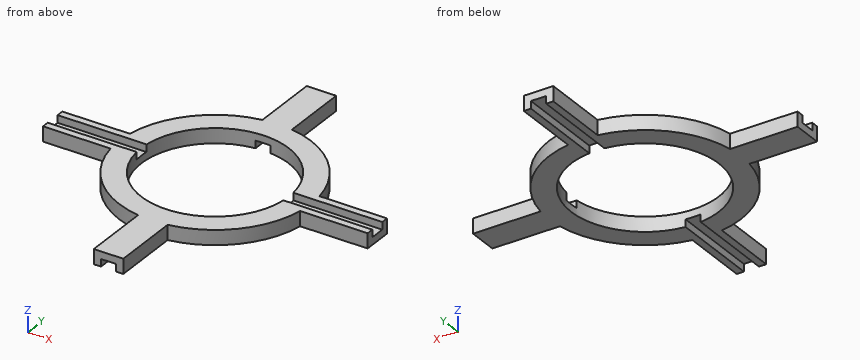
```python
from build123d import *

# Parameters (mm, degrees)
SKETCH1_R                    = 26
SKETCH1_R_2                  = 20
RELIEVED_FLOATING_RING_DEPTH = 4
SKETCH2_W                    = 20
SKETCH2_H                    = 8
X_SLIDE_PAD_1_DEPTH          = 4
SKETCH3_W                    = 8
SKETCH3_H                    = 20
Y_SLIDE_PAD_1_DEPTH          = 4
SKETCH4_W                    = 20
SKETCH4_H                    = 8
X_SLIDE_PAD_1_2_DEPTH        = 4
SKETCH5_W                    = 8
SKETCH5_H                    = 20
Y_SLIDE_PAD_1_2_DEPTH        = 4
SKETCH6_W                    = 4.1
SKETCH6_H                    = 90
LOWER_Y_SLOTS_W4P1_H2_DEPTH  = 2
SKETCH7_W                    = 90
SKETCH7_H                    = 4.1
UPPER_X_SLOTS_W4P1_H2_DEPTH  = 2


with BuildPart() as part:
    # Sketch1 → Relieved_Floating_Ring (new body)
    with BuildSketch(Plane.XY):
        Circle(SKETCH1_R)
        Circle(SKETCH1_R_2, mode=Mode.SUBTRACT)
    extrude(amount=RELIEVED_FLOATING_RING_DEPTH)

    # Sketch2 → X_Slide_Pad_-1 (add)
    with BuildSketch(Plane.XY):
        with Locations((-34, 0)):
            Rectangle(SKETCH2_W, SKETCH2_H)
    extrude(amount=X_SLIDE_PAD_1_DEPTH)

    # Sketch3 → Y_Slide_Pad_-1 (add)
    with BuildSketch(Plane.XY):
        with Locations((0, -34)):
            Rectangle(SKETCH3_W, SKETCH3_H)
    extrude(amount=Y_SLIDE_PAD_1_DEPTH)

    # Sketch4 → X_Slide_Pad_1 2 (add)
    with BuildSketch(Plane.XY):
        with Locations((34, 0)):
            Rectangle(SKETCH4_W, SKETCH4_H)
    extrude(amount=X_SLIDE_PAD_1_2_DEPTH)

    # Sketch5 → Y_Slide_Pad_1 2 (add)
    with BuildSketch(Plane.XY):
        with Locations((0, 34)):
            Rectangle(SKETCH5_W, SKETCH5_H)
    extrude(amount=Y_SLIDE_PAD_1_2_DEPTH)

    # Sketch6 → Lower_Y_Slots_W4p1_H2 (cut)
    with BuildSketch(Plane(origin=(0, 0, 0), x_dir=(-1, 0, 0), z_dir=(0, 0, -1))):
        Rectangle(SKETCH6_W, SKETCH6_H)
    extrude(amount=-LOWER_Y_SLOTS_W4P1_H2_DEPTH, mode=Mode.SUBTRACT)

    # Sketch7 → Upper_X_Slots_W4p1_H2 (cut)
    with BuildSketch(Plane.XY.offset(4)):
        Rectangle(SKETCH7_W, SKETCH7_H)
    extrude(amount=-UPPER_X_SLOTS_W4P1_H2_DEPTH, mode=Mode.SUBTRACT)


solid = part.part
```
Geometry: final body of the model. Coordinates: model frame, mm. Coordinates: 2 decimals unless noted, no trailing zeros. Write each loop counter-clockwise with the first axis right and the second up, starting at its lowest first coordinate (ties: lowest second). Pieces come first, ordered by that corner, then holes. Notation, with made-up numbers: M 7,70 L 35,70 A8 cw 35,75 Z; hole C 19,-29 d11. An arc over 180 degrees is marked long. Use CSV: the item, a comma, the result in double quotes. Start each with the question number.
1. Cut plane D-D on x = -37. Return the cut outline in (y, z).
2. Cut plane C-C on x = 0. Return the cut outline in (y, z).
3. Ray query, probe 1 along Y at (x, z) = (0, 2.3); probe 2 along X at (y, z) = (-28, 1.95). Return the intervals inside material, ascending.
4. Cut plane A-A on y = 0. Return the cut outline in (x, z), plus the area to 3 significant figures.
5. Cut plane B-B on z = 0.95. Return the cut outline in (x, y).
6. First-contact query: P1, Ø0.6, axis at x = -33.5, z = 2.5, coming from the -Y side; P2, Ø2, axis at x = 0, y = 30, coming from the -Z side; P3, Ø1, axis at y = -37.5, z = 0.5, coming from the +X side; P4, Ø2, axis at x = 16, y = 7, coming from the -Z side. Flat tips, straight axial feed; report the tip coordinate or a pass-through.
Entries:
1,outline,"M -4,0 L 4,0 L 4,4 L 2.05,4 L 2.05,2 L -2.05,2 L -2.05,4 L -4,4 Z"
2,outline,"M -44,2 L -20,2 L -20,4 L -44,4 Z; M 20,2 L 44,2 L 44,4 L 20,4 Z"
3,probe 1,"-44 to -20, 20 to 44"
3,probe 2,"-4 to -2.05, 2.05 to 4"
4,outline,"M -44,0 L -20,0 L -20,2 L -44,2 Z; M 20,0 L 44,0 L 44,2 L 20,2 Z"
4,area,"96.0 mm²"
5,outline,"M -44,-4 L -25.69,-4 A26 ccw -4,-25.69 L -4,-44 L -2.05,-44 L -2.05,-19.89 A20 cw -2.05,19.89 L -2.05,44 L -4,44 L -4,25.69 A26 ccw -25.69,4 L -44,4 Z; M 2.05,-44 L 4,-44 L 4,-25.69 A26 ccw 25.69,-4 L 44,-4 L 44,4 L 25.69,4 A26 ccw 4,25.69 L 4,44 L 2.05,44 L 2.05,19.89 A20 cw 2.05,-19.89 Z"
6,P1,"y = -4"
6,P2,"z = 2"
6,P3,"x = 4"
6,P4,"through"
